```python
from build123d import *

# Parameters (mm, degrees)
SKETCH1_W           = 75
SKETCH1_H           = 3
CHAMFER1_SIZE       = 0.4
TAPPED_HOLE10_D     = 2.5
TAPPED_HOLE10_DEPTH = 8.5
TAPPED_HOLE10_TIP   = 0.751075774
TAPPED_HOLE11_D     = 2.5
TAPPED_HOLE11_DEPTH = 8.5
TAPPED_HOLE11_TIP   = 0.751075774


with BuildPart() as part:
    # Sketch1 → Revolve1 (revolve)
    with BuildSketch(Plane.XY, mode=Mode.PRIVATE) as revolve1_sk:
        with Locations((37.5, 1.5)):
            Rectangle(SKETCH1_W, SKETCH1_H)
    revolve(revolve1_sk.sketch.rotate(Axis((0, 0, 0), (1, 0, 0)), 90), axis=Axis((0, 0, 0), (1, 0, 0)))

    # Chamfer1
    chamfer1_edges = [part.edges().sort_by_distance(p)[0] for p in [
        (0, 0, -3),
        (75, 0, -3),
    ]]
    chamfer(chamfer1_edges, length=CHAMFER1_SIZE)

    # Tapped Hole10
    with Locations(Plane.ZY):
        with Locations((0, 0)):
            Hole(TAPPED_HOLE10_D / 2, depth=TAPPED_HOLE10_DEPTH)
            with Locations((0, 0, -(TAPPED_HOLE10_DEPTH + TAPPED_HOLE10_TIP / 2))):  # 118° drill point
                Cone(0, TAPPED_HOLE10_D / 2, TAPPED_HOLE10_TIP, mode=Mode.SUBTRACT)

    # Tapped Hole11
    with Locations(Plane(origin=(75, 0, 0), x_dir=(0, 0, -1), z_dir=(1, 0, 0))):
        with Locations((0, 0)):
            Hole(TAPPED_HOLE11_D / 2, depth=TAPPED_HOLE11_DEPTH)
            with Locations((0, 0, -(TAPPED_HOLE11_DEPTH + TAPPED_HOLE11_TIP / 2))):  # 118° drill point
                Cone(0, TAPPED_HOLE11_D / 2, TAPPED_HOLE11_TIP, mode=Mode.SUBTRACT)


solid = part.part
```
The model under review builds one solid part; all positions refer to its coordinate system, in mm. A direction names the side the tool comes from. Give positions to 0.01 mm unless a question says otherwise; leave off trailing zeros. Order: outer loops, then holes, each group sorted by start corner. A loop starts at its lowest first (then second) coordinate and runs counter-clockwise, first axis right, second up. Notation, with made-up numbers: (48.25, 53.25) - (52.25, 53.25) arc R25 ccw to (52.25, 92.25) - close; hole circle Ø1 at (55, -2.75). An arc over 180 degrees is marked (long way). Use CSV: the item, a comma, the result in double quotes. Start each with the question number.
Q1. We need section A-A, the plane x = 19. Write out the cut boundary in (y, z), and give its area (3 significant figures).
Q2. To check wall thickness, follow line 1 along Y through (x, z) = (2.5, 0); line 2 along Z through (x, y) = (49, 0.2); line 3 along Y through (x, z) = (20.5, 1.15). State the ranges of each line that lie inside material, in increasing order. Write a range as [from, to].
Q3. The part is to be moulded in two halves that separate along Y. For faces 4 (the conical face through (65.88, -0.21, 0.05)), 5 (the flat face through (0, 1, 1)), 6 (the conical face through (9.12, -0.21, -0.05)), 7 (the cylindrical face through (38.02, -0.9, 2.86)), say which applies: +Y half, -Y half, draft (parallel to the pull), parting line (faces both ways), or undercut.
Q4. We need section B-B, the plane x = 70. Write out the cut boundary in (y, z).
Q5. Clearance check with flat-ended pins moving along their axes: pin 1 Ø3 at (y, z) = (0, 0) entering from +X; pin 2 Ø1.5 at (x, z) = (36.5, 1) entering from +Y; pin 3 Ø1.5 at (x, z) = (8, -1) entering from -Y; pin 4 Ø2 at (x, y) = (67, -2) entering from +Z. State where each tip first meets the part, or that it passes through.
Q6. Tool access review of faces 1 (the cylindrical face through (4.31, -1.22, 0.27)), 2 (the flat face through (75, 1, 1)), 3 (the cylindrical face through (70.69, -1.22, -0.27)): name each direction out of +Z, -Z, +X, -X, +Y, -Y from which nothing blocks a thin tool from reaching the whole face with its end or side.
Outcome:
1,outline,"circle Ø6 at (0, 0)"
1,area,"28.3 mm^2"
2,line 1,"y = [-3, -1.25], [1.25, 3]"
2,line 2,"z = [-2.99, 2.99]"
2,line 3,"y = [-2.77, 2.77]"
3,face 4,"undercut"
3,face 5,"draft"
3,face 6,"undercut"
3,face 7,"parting line"
4,outline,"circle Ø6 at (0, 0); hole circle Ø2.5 at (0, 0)"
5,pin 1,"stops at x = 75"
5,pin 2,"stops at y = 2.99"
5,pin 3,"stops at y = -2.99"
5,pin 4,"stops at z = 2.83"
6,face 1,"-X"
6,face 2,"+Z, -Z, +X, +Y, -Y"
6,face 3,"+X"
